Check sheet for the modelled part. Datum: model origin and axes. Units: mm. Round coordinates to 2 decimals unless told otherwise and drop trailing zeros. Write each loop counter-clockwise with the first axis right and the second up, starting at its lowest first coordinate (ties: lowest second). Pieces come first, ordered by that corner, then holes. Notation, with made-up numbers: (70.25, 47) -> (83.25, 47) arc R19 cw to (83.25, 63) -> close; hole circle Ø11 at (-4, -37). An arc over 180 degrees is marked (long way). Answer as a JSON object with one key per item and string values. Group by question number.
```python
from build123d import *

# Parameters (mm, degrees)
SKETCH_1_W          = 15
SKETCH_1_H          = 66.8
SKETCH_1_R          = 1.6
SKETCH_1_R_2        = 1.25
SKETCH_1_R_3        = 0.8
EXTRUDE_1_DEPTH     = 3
SKETCH_1_5_R        = 2
SKETCH_1_5_R_2      = 1.3
CUT_EXTRUDE_3_DEPTH = 1.5


with BuildPart() as part:
    # Sketch 1 → Extrude 1 (new body)
    with BuildSketch(Plane(origin=(0, 0, 0), x_dir=(1, 0, 0), z_dir=(0, 1, 0))):
        with Locations((7.5, 1)):
            Rectangle(SKETCH_1_W, SKETCH_1_H)
        with BuildLine():
            ThreePointArc((10.488636323, -15.860869565), (7.5, -27.6), (4.511363677, -15.860869565))
            ThreePointArc((4.511363677, -15.860869565), (7.5, -12.6), (10.488636323, -15.860869565))
        make_face(mode=Mode.SUBTRACT)
        with Locations(Location((7.5, 23.35, 0), (0, 0, 270))):
            Circle(SKETCH_1_R, mode=Mode.SUBTRACT)
        with Locations(Location((3, -3, 0), (0, 0, 270))):
            Circle(SKETCH_1_R_2, mode=Mode.SUBTRACT)
        with Locations(Location((12, -3, 0), (0, 0, 270))):
            Circle(SKETCH_1_R_2, mode=Mode.SUBTRACT)
        with Locations(Location((3, -29.4, 0), (0, 0, 270))):
            Circle(SKETCH_1_R_2, mode=Mode.SUBTRACT)
        with Locations(Location((12, -29.4, 0), (0, 0, 270))):
            Circle(SKETCH_1_R_2, mode=Mode.SUBTRACT)
        with Locations(Location((3, 4.25, 0), (0, 0, 270))):
            Circle(SKETCH_1_R_3, mode=Mode.SUBTRACT)
        with Locations(Location((12, 4.25, 0), (0, 0, 270))):
            Circle(SKETCH_1_R_3, mode=Mode.SUBTRACT)
        with Locations(Location((3, 32.15, 0), (0, 0, 270))):
            Circle(SKETCH_1_R_3, mode=Mode.SUBTRACT)
        with Locations(Location((12, 32.15, 0), (0, 0, 270))):
            Circle(SKETCH_1_R_3, mode=Mode.SUBTRACT)
    extrude(amount=EXTRUDE_1_DEPTH)

    # Sketch 1_5 → Cut-Extrude 3 (cut)
    with BuildSketch(Plane(origin=(0, 0, 0), x_dir=(1, 0, 0), z_dir=(0, 1, 0))):
        with Locations(Location((3, -3, 0), (0, 0, 270))):
            Circle(SKETCH_1_5_R)
        with Locations(Location((12, -3, 0), (0, 0, 270))):
            Circle(SKETCH_1_5_R)
        with Locations(Location((3, -29.4, 0), (0, 0, 270))):
            Circle(SKETCH_1_5_R)
        with Locations(Location((12, -29.4, 0), (0, 0, 270))):
            Circle(SKETCH_1_5_R)
        with Locations(Location((3, 4.25, 0), (0, 0, 270))):
            Circle(SKETCH_1_5_R_2)
        with Locations(Location((12, 4.25, 0), (0, 0, 270))):
            Circle(SKETCH_1_5_R_2)
        with Locations(Location((3, 32.15, 0), (0, 0, 270))):
            Circle(SKETCH_1_5_R_2)
        with Locations(Location((12, 32.15, 0), (0, 0, 270))):
            Circle(SKETCH_1_5_R_2)
    extrude(amount=CUT_EXTRUDE_3_DEPTH, mode=Mode.SUBTRACT)


solid = part.part
```
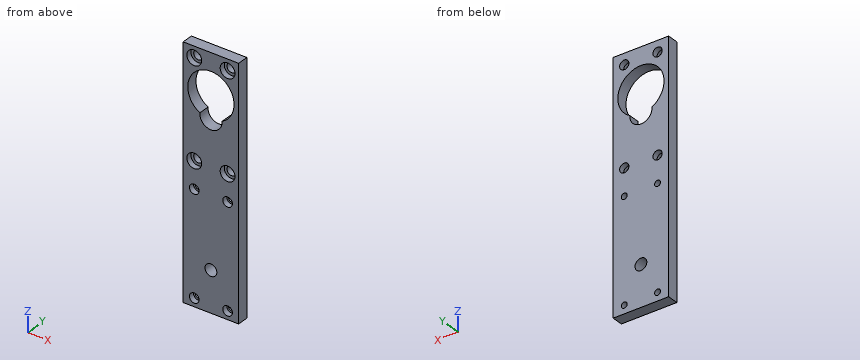
(1) Section check A-A on x = 7.5. Record the cut outline in (y, z).
(2) Section check B-B on z = -4.25. Record the cut outline in (x, y), then the cut area to 3 significant figures.
(3) Scan lines: line 1 along X through (y, z) = (2.4, -4.25); line 2 along X through (y, z) = (1, 3); line 3 along Z through (x, y) = (2.75, 0.45). Record each from-to range of solid material in increasing order.
(4) Section check C-C on z = 21.35. Record the cut outline in (x, y), then the cut area to 3 significant figures.
(5) Section check D-D on y = 0.85. State how many separate pieces and enclosed holes the cut face has, then the cut area to 3 significant figures.
(6) Go/stop test with flat-tipped pins: pin 1 Ø1.5 at (x, z) = (3, 3) entering from +Y; pin 2 Ø3 at (x, z) = (12, 29.4) entering from -Y. Record where each tip stops, or that it passes through.
Data:
{
 "1": {"outline": "(0, -34.4) -> (3, -34.4) -> (3, -24.95) -> (0, -24.95) -> close; (0, -21.75) -> (3, -21.75) -> (3, 12.6) -> (0, 12.6) -> close; (0, 27.6) -> (3, 27.6) -> (3, 32.4) -> (0, 32.4) -> close"},
 "2": {"outline": "(0, 0) -> (1.7, 0) -> (1.7, 1.5) -> (2.2, 1.5) -> (2.2, 3) -> (0, 3) -> close; (3.8, 1.5) -> (4.3, 1.5) -> (4.3, 0) -> (10.7, 0) -> (10.7, 1.5) -> (11.2, 1.5) -> (11.2, 3) -> (3.8, 3) -> close; (12.8, 1.5) -> (13.3, 1.5) -> (13.3, 0) -> (15, 0) -> (15, 3) -> (12.8, 3) -> close", "area": "32.4 mm²"},
 "3": {"line 1": "x = 0 to 2.2, 3.8 to 11.2, 12.8 to 15", "line 2": "x = 0 to 1, 5 to 10, 14 to 15", "line 3": "z = -34.4 to -33.43, -30.87 to -5.53, -2.97 to 1.02, 4.98 to 17.29, 25.41 to 27.42, 31.38 to 32.4"},
 "4": {"outline": "(0, 0) -> (1.25, 0) -> (1.25, 3) -> (0, 3) -> close; (13.75, 0) -> (15, 0) -> (15, 3) -> (13.75, 3) -> close", "area": "7.50 mm²"},
 "5": {"separate pieces": "1", "enclosed holes": "10", "area": "787 mm²"},
 "6": {"pin 1": "passes through", "pin 2": "stops at y = 1.5"}
}
